```python
from build123d import *

# Parameters (mm, degrees)
F1_DEPTH = 38.1
F2_SIZE  = 5.08
F3_SIZE  = 5.08
F4_SIZE  = 5.08
F5_SIZE  = 5.08
F6_SIZE  = 5.08


# Not quite as in the source:
# - the program builds the solid bodies; features that only make, move or delete a surface that nothing else refers to are left out


with BuildPart() as f1:
    # F0 (on Front) → F1 (new body)
    with BuildSketch(Plane.XZ):
        Polygon((5.5975063319, -72.0986601401), (65.238024426, -31.2017473888), (59.6405180942, 40.8969127513), (-5.5975063319, 72.0986601401), (-65.238024426, 31.2017473888), (-59.6405180942, -40.8969127513), align=None)
    extrude(amount=F1_DEPTH)

    # F2
    f2_edges = [f1.edges().sort_by_distance(p)[0] for p in [
        (27.021506, -38.1, 56.497786),
    ]]
    chamfer(f2_edges, length=F2_SIZE)

    # F3
    f3_edges = [f1.edges().sort_by_distance(p)[0] for p in [
        (62.666292, -38.1, 1.923443),
    ]]
    chamfer(f3_edges, length=F3_SIZE)

    # F4
    f4_edges = [f1.edges().sort_by_distance(p)[0] for p in [
        (-62.439271, 0, -4.847583),
        (62.439271, 0, 4.847583),
        (-27.021506, 0, -56.497786),
        (32.998896, -38.1, -53.30888),
        (-35.417765, 0, 51.650204),
        (-27.021506, -38.1, -56.497786),
        (27.021506, 0, 56.497786),
        (-62.439271, -38.1, -4.847583),
        (35.417765, 0, -51.650204),
        (-37.836635, -38.1, 49.991528),
    ]]
    chamfer(f4_edges, length=F4_SIZE)

    # F5
    f5_edges = [f1.edges().sort_by_distance(p)[0] for p in [
        (5.597506, -19.05, -72.09866),
    ]]
    chamfer(f5_edges, length=F5_SIZE)

    # F6
    f6_edges = [f1.edges().sort_by_distance(p)[0] for p in [
        (-5.597506, -19.05, 72.09866),
        (-65.238024, -19.05, 31.201747),
        (65.238024, -19.05, -31.201747),
        (59.640518, -19.05, 40.896913),
    ]]
    chamfer(f6_edges, length=F6_SIZE)


solid = f1.part
```
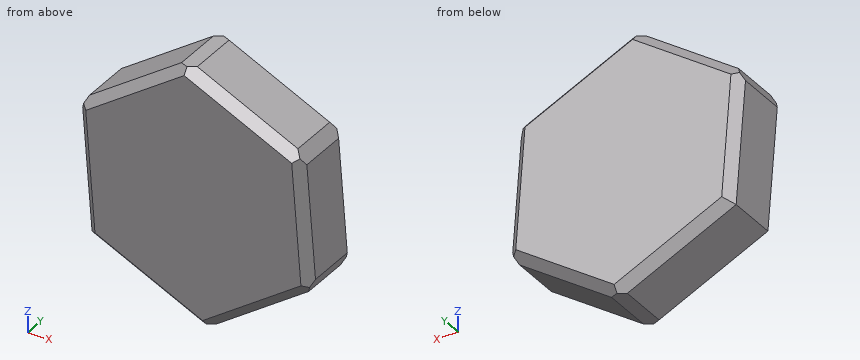
Verification items for the finished model (mm, model axes). Coordinates: 2 decimals unless noted, no trailing zeros. Loops run counter-clockwise (first coordinate to the right, second up) from the corner with the lowest first, then second, coordinate; pieces in that order, holes last. Notation, with made-up numbers: (27.5, 26) -> (63.5, 26) arc R28 ccw to (63.5, 47) -> close; hole circle Ø5 at (79.25, 59.5). An arc over 180 degrees is marked (long way). Answer in a Markdown table with one row per item.
1) Depth check by flat-ended pin: P1, Ø8, axis at y = -12.5, z = 9.5, coming from the -X side; P2, Ø5, axis at y = -7.5, z = 55, coming from the -X side; P3, Ø1, axis at x = 22, y = -31, coming from the -Z side. Enter the tip coordinate at first touch or a pass-through.
The answers:
| item | result |
|---|---|
| P1 | stops at x = -63.86 |
| P2 | stops at x = -34.18 |
| P3 | stops at z = -61.19 |
2) Scan lines: line 1 along X through (y, z) = (-1.5, 43.5); line 2 along Z through (x, y) = (-38, -2.5); line 3 along Z through (x, y) = (-36.5, -33.5). Record each from-to range of solid material in increasing order. Write a range as from..to.
The answers:
| item | result |
|---|---|
| line 1 | x = -40.97..45.9 |
| line 2 | z = -48.39..46.75 |
| line 3 | z = -51.43..50.33 |
3) Section check C-C (z = 19). Record the cut outline in (x, y).
The answers:
| item | result |
|---|---|
| outline | (-64.29, -33.02) -> (-59.2, -38.1) -> (56.25, -38.1) -> (61.34, -33.02) -> (61.34, -5.08) -> (56.25, 0) -> (-59.2, 0) -> (-64.29, -5.08) -> close |
4) Section check B-B (x = 33). Record the cut outline in (y, z), and give its area (3 significant figures).
The answers:
| item | result |
|---|---|
| outline | (-38.1, -47.15) -> (-33.02, -53.31) -> (-5.08, -53.31) -> (0, -47.15) -> (0, 48.01) -> (-5.08, 53.64) -> (-33.02, 53.64) -> (-38.1, 48.01) -> close |
| area | 4,010 mm2 |
5) Section check A-A (y = -15). Record the cut outline in (x, z).
The answers:
| item | result |
|---|---|
| outline | (-64.84, 26.14) -> (-59.64, -40.9) -> (1.01, -69.91) -> (9.79, -69.23) -> (61.05, -34.07) -> (64.84, -26.14) -> (60.03, 35.83) -> (55.06, 43.09) -> (-1.01, 69.91) -> (-9.79, 69.23) -> (-61.05, 34.07) -> close |
